Read the model definition and answer for the solid it produces. Units are mm, in the model's axes. Face numbers are marked on the shaded views. Give positions to 0.01 mm unless a question says otherwise; leave off trailing zeros. Write each loop counter-clockwise with the first axis right and the second up, starting at its lowest first coordinate (ties: lowest second). Pieces come first, ordered by that corner, then holes. Notation, with made-up numbers: (-9.75, -26) -> (48.25, -26) arc R21 ccw to (48.25, -12) -> close; hole circle Ø10 at (-25.75, 82.5). An arc over 180 degrees is marked (long way). Answer as CSV lines item,"result". Start each with the question number.
1. The part is cut by section C-C, the plane z = -59. Determine the outline of the cut face in (x, y).
2. The part is cut by section A-A, the plane y = 0. Determine the outline of the cut face in (x, z) (3 decimals), and give its area (3 significant figures).
3. Given pin 1 (5 mm diameter, centred on x = -6, z = -84.5, fed in from +Y); pin 2 (13 mm diameter, centred on x = 0, y = -50.8, fed in from -Z); pin 3 (6 mm diameter, centred on y = 128.5, z = -28.5, fed in from -X), each flat-ended and moving along its own axis, determine where each tip first touches the part or whether it passes through.
4. Find the intervals of material crossed by line 1 (Y direction, x = 0, z = 1); line 2 (X direction, y = -1, z = -22); line 3 (Y direction, x = 50, z = 2), in increasing order.
5. The part is cut by section D-D, the plane y = -50.8. Determine the outline of the cut face in (x, z) (3 decimals).
6. For a pull along X with two mould halves and no side action, classify the marked faces 1, 2 and 3 as pulls with the +X half, pulls with the -X half, needs draft (parallel to the pull), parting line crosses it, or undercut.
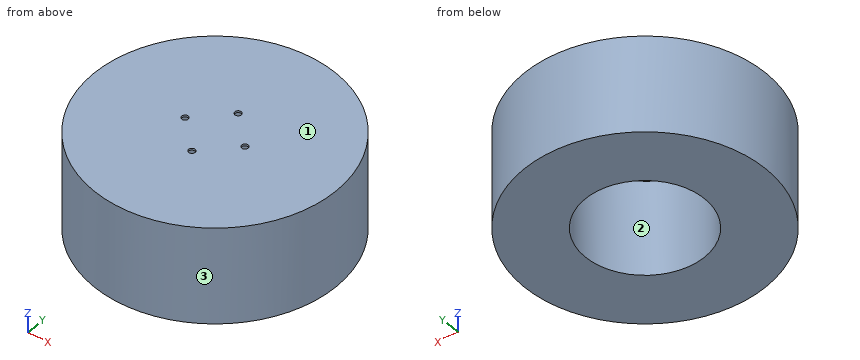
from build123d import *

# Parameters (mm, degrees)
SKETCH1_R           = 101.6
SKETCH1_R_2         = 5.55625
BOSS_EXTRUDE2_DEPTH = 3.175
SKETCH2_R           = 205.74
SKETCH2_R_2         = 101.6
BOSS_EXTRUDE3_DEPTH = 165.1


with BuildPart() as part:
    # Sketch1 → Boss-Extrude2 (new body)
    with BuildSketch(Plane.XY):
        Circle(SKETCH1_R)
        with Locations((0, 50.8)):
            Circle(SKETCH1_R_2, mode=Mode.SUBTRACT)
        with Locations((50.8, 0)):
            Circle(SKETCH1_R_2, mode=Mode.SUBTRACT)
        with Locations((0, -50.8)):
            Circle(SKETCH1_R_2, mode=Mode.SUBTRACT)
        with Locations((-50.8, 0)):
            Circle(SKETCH1_R_2, mode=Mode.SUBTRACT)
    extrude(amount=BOSS_EXTRUDE2_DEPTH)

    # Sketch2 → Boss-Extrude3 (add)
    with BuildSketch(Plane.XY.offset(3.175)):
        Circle(SKETCH2_R)
        Circle(SKETCH2_R_2, mode=Mode.SUBTRACT)
    extrude(amount=-BOSS_EXTRUDE3_DEPTH)


solid = part.part
Results found:
1,outline,"circle Ø411.48 at (0, 0); hole circle Ø203.2 at (0, 0)"
2,outline,"(-205.74, -161.925) -> (-101.6, -161.925) -> (-101.6, 0) -> (-56.356, 0) -> (-56.356, 3.175) -> (-205.74, 3.175) -> close; (-45.244, 0) -> (45.244, 0) -> (45.244, 3.175) -> (-45.244, 3.175) -> close; (56.356, 0) -> (101.6, 0) -> (101.6, -161.925) -> (205.74, -161.925) -> (205.74, 3.175) -> (56.356, 3.175) -> close"
2,area,"35,000 mm²"
3,pin 1,"stops at y = 205.71"
3,pin 2,"stops at z = 0"
3,pin 3,"stops at x = -163.03"
4,line 1,"y = -205.74 to -56.36, -45.24 to 45.24, 56.36 to 205.74"
4,line 2,"x = -205.74 to -101.6, 101.6 to 205.74"
4,line 3,"y = -199.57 to -5.5, 5.5 to 199.57"
5,outline,"(-199.37, -161.925) -> (-87.988, -161.925) -> (-87.988, 0) -> (-5.556, 0) -> (-5.556, 3.175) -> (-199.37, 3.175) -> close; (5.556, 0) -> (87.988, 0) -> (87.988, -161.925) -> (199.37, -161.925) -> (199.37, 3.175) -> (5.556, 3.175) -> close"
6,face 1,"needs draft"
6,face 2,"undercut"
6,face 3,"parting line crosses it"
